Read the model definition and answer for the solid it produces. Units are mm, in the model's axes. Give positions to 0.01 mm unless a question says otherwise; leave off trailing zeros. Loops run counter-clockwise (first coordinate to the right, second up) from the corner with the lowest first, then second, coordinate; pieces in that order, holes last. Notation, with made-up numbers: (58, -3.5) -> (66, -3.5) arc R5 ccw to (66, 5.5) -> close; hole circle Ø11 at (66.25, -18.5). An arc over 180 degrees is marked (long way). Return JSON: item names as keys, results as strings. Group by question number.
from build123d import *

# Parameters (mm, degrees)
F2_R      = 113.5
F3_DEPTH  = 5
F4_R      = 1
F5_W      = 8
F5_H      = 18
F5_R      = 2.5
F7_DEPTH  = 12.5
F6_W      = 8
F6_H      = 18
F6_R      = 1.75
F8_DEPTH  = 12.5
F9_W      = 250
F9_H      = 100
F10_DEPTH = 150
F11_R     = 2
F12_R     = 2


with BuildPart() as f1:
    # F0 (on Front) → F1 (revolve)
    with BuildSketch(Plane.XZ):
        with BuildLine():
            Line((-114.5, -3), (-106.5, -3))
            Line((-106.5, -3), (-106.5, 0))
            Line((-106.5, 0), (-106.5, 7))
            Line((-106.5, 7), (-106.888494173, 7))
            Line((-106.888494173, 7), (-118.388494173, 7))
            Line((-118.388494173, 7.0000000475), (-118.388494173, 1.0000000475))
            ThreePointArc((-118.388494173, 1.0000000475), (-116.9832708565, -1.8549081567), (-116.5, -5))
            Line((-116.5, -5), (-116.5, -11))
            Line((-116.5, -11), (-114.5, -11))
            Line((-114.5, -11), (-114.5, -3))
        make_face()
    revolve(axis=Axis((0, 0, -0.2650997043), (0, 0, 1)))

    # F2 (on Top) → F3 (cut)
    with BuildSketch(Plane.XY):
        Circle(F2_R)
    extrude(amount=F3_DEPTH, mode=Mode.SUBTRACT)

    # F4
    f4_edges = [f1.edges().sort_by_distance(p)[0] for p in [
        (116.5, 0, -11),
    ]]
    fillet(f4_edges, radius=F4_R)

    # F5 (on Front) → F7 (join, symmetric)
    with BuildSketch(Plane.XZ):
        with Locations((-119.7, -2)):
            Rectangle(F5_W, F5_H)
        with Locations((-119.2, -2)):
            Circle(F5_R, mode=Mode.SUBTRACT)
    extrude(amount=F7_DEPTH, both=True)

    # F6 (on Front) → F8 (join, symmetric)
    with BuildSketch(Plane.XZ):
        with Locations((119.7, -2)):
            Rectangle(F6_W, F6_H)
        with Locations((119.2, -2)):
            Circle(F6_R, mode=Mode.SUBTRACT)
    extrude(amount=F8_DEPTH, both=True)

    # F9 (on Front) → F10 (cut)
    with BuildSketch(Plane.XZ):
        with Locations((0.1239156971, -32.2915658355)):
            Rectangle(F9_W, F9_H)
    extrude(amount=-F10_DEPTH, mode=Mode.SUBTRACT)

    # F11
    f11_edges = [f1.edges().sort_by_distance(p)[0] for p in [
        (0, -113.5, 0),
    ]]
    fillet(f11_edges, radius=F11_R)

    # F12
    f12_edges = [f1.edges().sort_by_distance(p)[0] for p in [
        (123.7, -6.25, -11),
        (-123.7, -6.25, -11),
    ]]
    fillet(f12_edges, radius=F12_R)


solid = f1.part
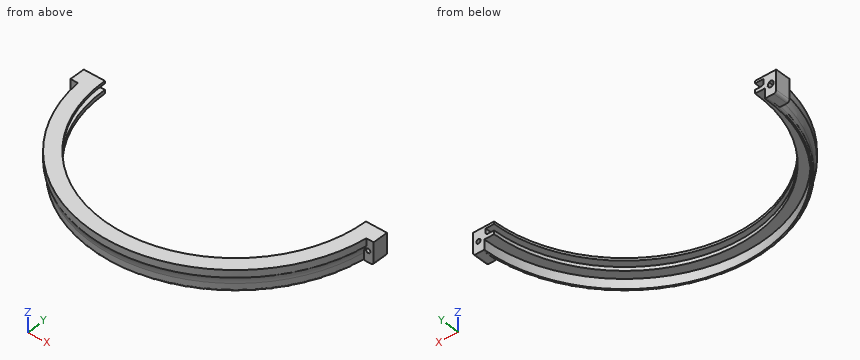
1. Section A-A on x = 0 is taken. Determine the outline of the cut face in (y, z), then the cut area to 3 significant figures.
2. Straight lines are drawn through the part: line 1 (Z direction, x = 119.2, y = -10); line 2 (Z direction, x = -119.2, y = -2.5); line 3 (X direction, y = -5, z = -2). For each, find the intervals that lie inside material, in ascending order. Write a range as from..to.
3. Flat-ended cylindrical pins translate along their axes: pin 1 Ø2 at (x, z) = (119.2, -2) entering from -Y; pin 2 Ø8 at (y, z) = (-49, 1) entering from +X; pin 3 Ø4 at (y, z) = (-95, 3.5) entering from +X; pin 4 Ø2 at (x, z) = (35, -8.5) entering from +Y. Find the tip coordinate at first contact, or state that the pin passes through.
Completed:
{
 "1": {"outline": "(-118.39, 1) arc R10.48 cw to (-116.5, -5) -> (-116.5, -10) arc R1 ccw to (-115.5, -11) -> (-114.5, -11) -> (-114.5, -3) -> (-106.5, -3) -> (-106.5, 0) -> (-111.5, 0) arc R2 cw to (-113.5, 2) -> (-113.5, 5) -> (-106.5, 5) -> (-106.5, 7) -> (-118.39, 7) -> close", "area": "96.6 mm²"},
 "2": {"line 1": "z = -11..-3.75, -0.25..7", "line 2": "z = -11..-4.5, 0.5..7", "line 3": "x = -123.7..-121.7, -116.83..-106.38, 106.38..117.45, 120.95..123.7"},
 "3": {"pin 1": "passes through", "pin 2": "stops at x = 109.5", "pin 3": "stops at x = 73.26", "pin 4": "stops at y = -108.69"}
}
